```python
from build123d import *

# Parameters (mm, degrees)
CROQUIS1_W              = 43
CROQUIS1_H              = 24
SALIENTE_EXTRUIR1_DEPTH = 1.4
CROQUIS2_R              = 0.983927781
CROQUIS2_R_2            = 0.985
SALIENTE_EXTRUIR2_DEPTH = 0.05
CROQUIS3_W              = 0.64
CROQUIS3_H              = 0.64
CORTAR_EXTRUIR1_DEPTH   = 1.81
CROQUIS4_R              = 0.385
CORTAR_EXTRUIR2_DEPTH   = 1.81
CROQUIS5_W              = 34.338370929
CROQUIS5_H              = 21.924969232
SALIENTE_EXTRUIR3_DEPTH = 2.39
REDONDEO1_R             = 0.4


with BuildPart() as part:
    # Croquis1 → Saliente-Extruir1 (new body)
    with BuildSketch(Plane(origin=(0, 0, 0), x_dir=(1, 0, 0), z_dir=(0, 1, 0))):
        Rectangle(CROQUIS1_W, CROQUIS1_H)
    extrude(amount=SALIENTE_EXTRUIR1_DEPTH)

    # Croquis2 → Saliente-Extruir2 (add)
    with BuildSketch(Plane(origin=(0, 1.4, 0), x_dir=(1, 0, 0), z_dir=(0, 1, 0))):
        with Locations((-20.02, 7.64)):
            Circle(CROQUIS2_R)
        with Locations((-20.02, 5.1)):
            Circle(CROQUIS2_R)
        with Locations((-20.02, 2.56)):
            Circle(CROQUIS2_R)
        with Locations((-20.02, 0.02)):
            Circle(CROQUIS2_R)
        with Locations((-20.02, -2.52)):
            Circle(CROQUIS2_R)
        with Locations((-20.02, -5.06)):
            Circle(CROQUIS2_R)
        with Locations((-20.02, -7.6)):
            Circle(CROQUIS2_R)
        with Locations((18.5, 7.82)):
            Circle(CROQUIS2_R_2)
        with Locations((18.5, 5.28)):
            Circle(CROQUIS2_R_2)
        with Locations((18.5, 2.74)):
            Circle(CROQUIS2_R_2)
        with Locations((18.5, 0.2)):
            Circle(CROQUIS2_R_2)
    extrude(amount=SALIENTE_EXTRUIR2_DEPTH)

    # Croquis3 → Cortar-Extruir1 (cut)
    with BuildSketch(Plane(origin=(0, 1.45, 0), x_dir=(1, 0, 0), z_dir=(0, 1, 0))):
        with Locations((-20.02, 5.1)):
            Rectangle(CROQUIS3_W, CROQUIS3_H)
        with Locations((-20.02, 7.64)):
            Rectangle(CROQUIS3_W, CROQUIS3_H)
        with Locations((-20.02, 2.56)):
            Rectangle(CROQUIS3_W, CROQUIS3_H)
        with Locations((-20.02, 0.02)):
            Rectangle(CROQUIS3_W, CROQUIS3_H)
        with Locations((-20.02, -2.52)):
            Rectangle(CROQUIS3_W, CROQUIS3_H)
        with Locations((-20.02, -5.06)):
            Rectangle(CROQUIS3_W, CROQUIS3_H)
        with Locations((-20.02, -7.6)):
            Rectangle(CROQUIS3_W, CROQUIS3_H)
    extrude(amount=-CORTAR_EXTRUIR1_DEPTH, mode=Mode.SUBTRACT)

    # Croquis4 → Cortar-Extruir2 (cut)
    with BuildSketch(Plane(origin=(0, 1.45, 0), x_dir=(1, 0, 0), z_dir=(0, 1, 0))):
        with Locations((18.5, 5.28)):
            Circle(CROQUIS4_R)
        with Locations((18.5, 7.82)):
            Circle(CROQUIS4_R)
        with Locations((18.5, 2.74)):
            Circle(CROQUIS4_R)
        with Locations((18.5, 0.2)):
            Circle(CROQUIS4_R)
    extrude(amount=-CORTAR_EXTRUIR2_DEPTH, mode=Mode.SUBTRACT)

    # Croquis5 → Saliente-Extruir3 (add)
    with BuildSketch(Plane(origin=(0, 1.4, 0), x_dir=(1, 0, 0), z_dir=(0, 1, 0))):
        with Locations((-0.967278054, -0.120909757)):
            Rectangle(CROQUIS5_W, CROQUIS5_H)
    extrude(amount=SALIENTE_EXTRUIR3_DEPTH)

    # Redondeo1
    redondeo1_edges = [part.edges().sort_by_distance(p)[0] for p in [
        (-18.136463519, 2.595, -10.841574859),
        (-18.136463519, 2.595, 11.083394373),
        (16.20190741, 2.595, 11.083394373),
        (16.20190741, 2.595, -10.841574859),
        (-18.136463519, 3.79, 0.120909757),
        (-0.967278054, 3.79, 11.083394373),
        (16.20190741, 3.79, 0.120909757),
        (-0.967278054, 3.79, -10.841574859),
    ]]
    fillet(redondeo1_edges, radius=REDONDEO1_R)


solid = part.part
```
Input: part model. Units: mm. Frame: model coordinates. A direction names the side the tool comes from. Round coordinates to 2 decimals unless told otherwise and drop trailing zeros. Write each loop counter-clockwise with the first axis right and the second up, starting at its lowest first coordinate (ties: lowest second). Pieces come first, ordered by that corner, then holes. Notation, with made-up numbers: (-6, -25.5) - (12, -25.5) arc R22 cw to (12, 3.5) - close; hole circle Ø7 at (67.25, 38). An arc over 180 degrees is marked (long way). Write item = value, one per line.
(1) Material intervals for probe 1 along X at (y, z) = (0.9, -5.28) (3 decimals); probe 2 along Z at (x, y) = (18.5, 0.85) (3 decimals); probe 3 along Z at (x, y) = (7.5, 1.9), sorted ascending.
Geometry check:
probe_1 = -21.5 to -20.34, -19.7 to 18.115, 18.885 to 21.5
probe_2 = -12 to -8.205, -7.435 to -5.665, -4.895 to -3.125, -2.355 to -0.585, 0.185 to 12
probe_3 = -10.84 to 11.08
(2) Access query for faces 1 (the flat face through (0, 0, 0)), 2 (the flat face through (-20.5, 1.45, 0)), 3 (the flat face through (-1, 2, -10.842)). Directions: +Z, -Z, +X, -X, +Y, -Y. A direction counts if a zero-diameter tool reaches every point of the face in a straight line with its end or side. Return the directions, or none.
Geometry check:
face_1 = +Z, -Z, +X, -X, -Y
face_2 = +Z, -Z, -X, +Y
face_3 = -Z, +X, -X, +Y
(3) Section query A-A on x = 1.5. Output: boundary loops of the cut face in (y, z), then the cut area to 3 significant figures.
Geometry check:
outline = (0, -12) - (1.4, -12) - (1.4, -10.84) - (3.39, -10.84) arc R0.4 ccw to (3.79, -10.44) - (3.79, 10.68) arc R0.4 ccw to (3.39, 11.08) - (1.4, 11.08) - (1.4, 12) - (0, 12) - close
area = 85.9 mm^2
(4) Contact query for flat-ended pins moving along their axis: pin 1 Ø4 at (x, z) = (7.5, 9) entering from -Y; pin 2 Ø1 at (x, z) = (-20, -7.5) entering from +Y; pin 3 Ø2 at (y, z) = (3, 8) entering from +X. Output: stop coordinate, or through.
Geometry check:
pin_1 = 0
pin_2 = 1.45
pin_3 = 16.2
